The listing builds one solid part. Answer for the finished solid, in the listing's coordinates (mm). Face numbers are marked on the shaded views. A direction names the side the tool comes from. Coordinates: 2 decimals unless noted, no trailing zeros. Put each result on its own line as item: value. Start each with the question number.
```python
from build123d import *

# Parameters (mm, degrees)
SKETCH1_R           = 5
SKETCH1_R_2         = 2.5
BOSS_EXTRUDE1_DEPTH = 4
FILLET1_R           = 0.25
FILLET2_R           = 0.25
SKETCH2_R           = 4.25
SKETCH2_R_2         = 3
CUT_EXTRUDE1_DEPTH  = 0.25
SKETCH3_R           = 4.25
SKETCH3_R_2         = 3
CUT_EXTRUDE2_DEPTH  = 0.25


with BuildPart() as part:
    # Sketch1 → Boss-Extrude1 (new body)
    with BuildSketch(Plane.XY):
        Circle(SKETCH1_R)
        Circle(SKETCH1_R_2, mode=Mode.SUBTRACT)
    extrude(amount=BOSS_EXTRUDE1_DEPTH)

    # Fillet1
    fillet1_edges = [part.edges().sort_by_distance(p)[0] for p in [
        (-5, 0, 0),
        (-5, 0, 4),
    ]]
    fillet(fillet1_edges, radius=FILLET1_R)

    # Fillet2
    fillet2_edges = [part.edges().sort_by_distance(p)[0] for p in [
        (-2.5, 0, 0),
        (-2.5, 0, 4),
    ]]
    fillet(fillet2_edges, radius=FILLET2_R)

    # Sketch2 → Cut-Extrude1 (cut)
    with BuildSketch(Plane.XY.offset(4)):
        Circle(SKETCH2_R)
        Circle(SKETCH2_R_2, mode=Mode.SUBTRACT)
    extrude(amount=-CUT_EXTRUDE1_DEPTH, mode=Mode.SUBTRACT)

    # Sketch3 → Cut-Extrude2 (cut)
    with BuildSketch(Plane(origin=(0, 0, 0), x_dir=(-1, 0, 0), z_dir=(0, 0, -1))):
        Circle(SKETCH3_R)
        Circle(SKETCH3_R_2, mode=Mode.SUBTRACT)
    extrude(amount=-CUT_EXTRUDE2_DEPTH, mode=Mode.SUBTRACT)


solid = part.part
```
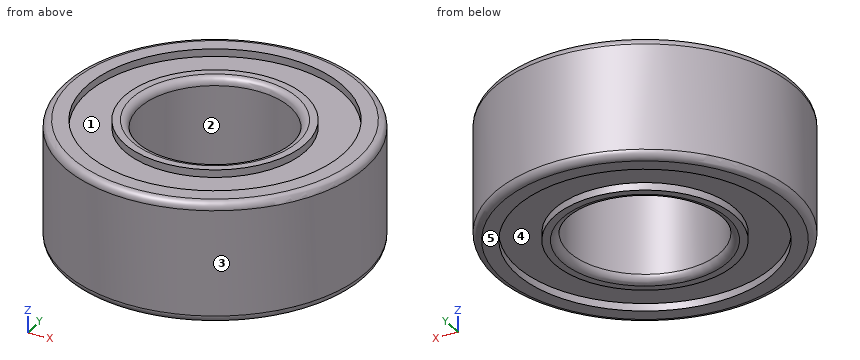
1) Straight lines are drawn through the part: probe 1 along Y at (x, z) = (0, 2.9); probe 2 along Y at (x, z) = (0, 0.15); probe 3 along Z at (x, y) = (-3.75, -1.25). For each, find the intervals that lie inside material, in ascending order.
2) Given pin 1 Ø3 at (x, y) = (0, 0) entering from +Z; pin 2 Ø1 at (x, z) = (3, 0.5) entering from +Y, each flat-ended and moving along its own axis, determine where each tip first touches the part or whether it passes through.
3) For the marked faces 1 and 2, determine the directions among +Z, -Z, +X, -X, +Y, -Y from which every point of the face is accessible in a straight line to the end or side of a thin tool.
4) Determine the mould class of the marked faces 3, 4 and 5 for opening direction X: +X half, -X half, draft (parallel to the pull), parting line (faces both ways), or undercut.
Answers follow:
1. probe 1: y = -5 to -2.5, 2.5 to 5
1. probe 2: y = -4.98 to -4.25, -3 to -2.52, 2.52 to 3, 4.25 to 4.98
1. probe 3: z = 0.25 to 3.75
2. pin 1: passes through
2. pin 2: stops at y = 4.33
3. face 1: +Z
3. face 2: +Z, -Z
4. face 3: parting line
4. face 4: undercut
4. face 5: draft
